Geometry check sheet. Reference: drawing and pictorial views, mm from the part's lowest x, y, z. A direction names the side the tool comes from. Coordinates: 2 decimals unless noted, no trailing zeros. Loops run counter-clockwise (first coordinate to the right, second up) from the corner with the lowest first, then second, coordinate; pieces in that order, holes last. Notation, with made-up numbers: (15.25, 50.25) - (71.25, 50.25) arc R19 cw to (71.25, 71.25) - close; hole circle Ø1 at (-12.75, 8). An arc over 180 degrees is marked (long way). One line per item, written item: value.
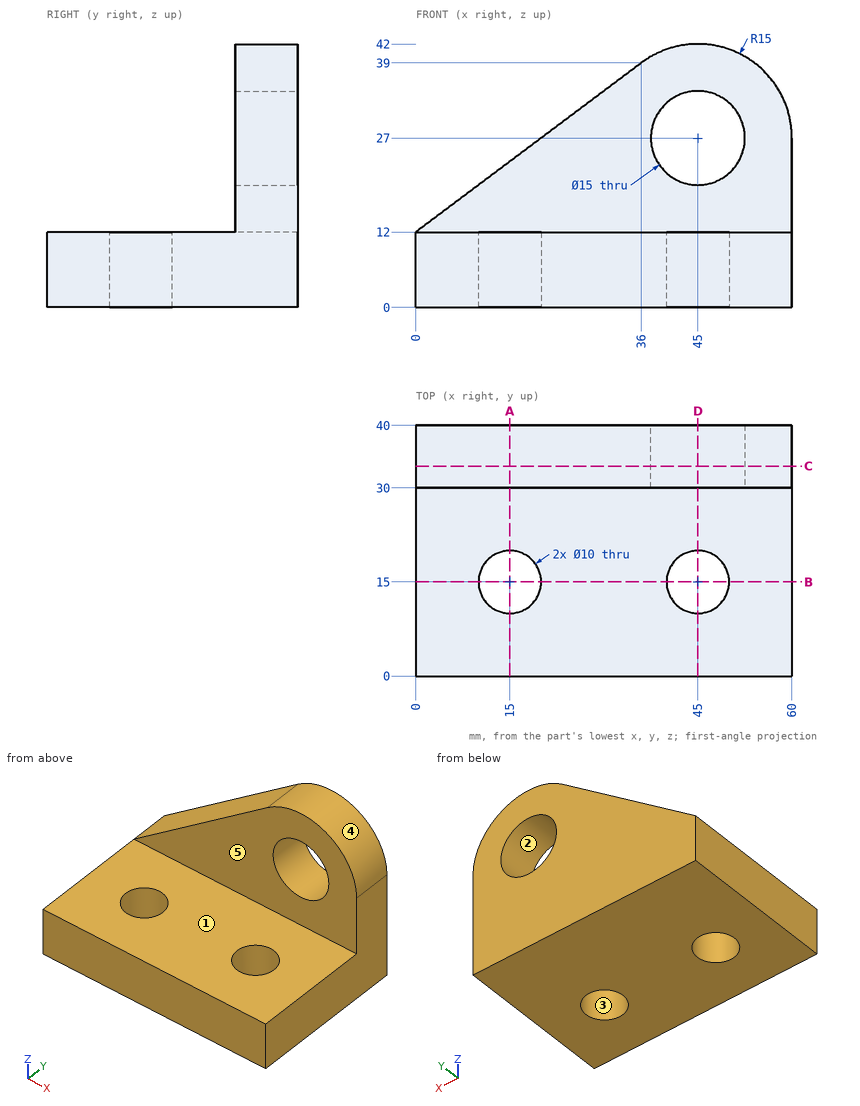
(1) Cross-section at C-C on y = 33.5. Record the cut outline in (x, z), and give its area (3 significant figures).
Reply:
outline: (0, 0) - (60, 0) - (60, 27) arc R15 ccw to (36, 39) - (0, 12) - close; hole circle Ø15 at (45, 27)
area: 1,690 mm2
(2) Access from +Z, -Z, +X, -X, +Y, -Y to the whole of each face (thin tool, end or side, straight path). Record for the marked faces 1 and 2.
Reply:
face 1: +Z, +X, -X, -Y
face 2: +Y, -Y
(3) Cross-section at D-D on x = 45. Record the cut outline in (y, z), and give its area (3 significant figures).
Reply:
outline: (0, 0) - (10, 0) - (10, 12) - (0, 12) - close; (20, 0) - (40, 0) - (40, 19.5) - (30, 19.5) - (30, 12) - (20, 12) - close; (30, 34.5) - (40, 34.5) - (40, 42) - (30, 42) - close
area: 510 mm2
(4) Release check for a two-part mould opening along X. For the marked faces 3, 4 and 5 record: pulls with the +X half, pulls with the -X half, needs draft (parallel to the pull), parting line crosses it, or undercut.
Reply:
face 3: undercut
face 4: parting line crosses it
face 5: needs draft
(5) Go/stop test with flat-tipped pins: pin 1 Ø9 at (x, z) = (45, 27) entering from +Y; pin 2 Ø2 at (y, z) = (29.5, 34.5) entering from -X; pin 3 Ø24 at (x, y) = (26, 20.5) entering from +Z; pin 4 Ø15 at (x, z) = (42.5, 21.5) entering from -Y. Record where each tip stops, or that it passes through.
Reply:
pin 1: through
pin 2: x = 28.85
pin 3: z = 37
pin 4: y = 30
(6) Material ranges on probe 1 along Y at (x, z) = (15, 7); probe 2 along Z at (x, y) = (45, 36); probe 3 along Y at (x, z) = (48, 39), recorded low to high. Write a range as from..to.
Reply:
probe 1: 0..10, 20..40
probe 2: 0..19.5, 34.5..42
probe 3: 30..40
(7) Cross-section at A-A on x = 15. Record the cut outline in (y, z).
Reply:
outline: (0, 0) - (10, 0) - (10, 12) - (0, 12) - close; (20, 0) - (40, 0) - (40, 23.25) - (30, 23.25) - (30, 12) - (20, 12) - close
(8) Cross-section at B-B on y = 15. Record the cut outline in (x, z).
Reply:
outline: (0, 0) - (10, 0) - (10, 12) - (0, 12) - close; (20, 0) - (40, 0) - (40, 12) - (20, 12) - close; (50, 0) - (60, 0) - (60, 12) - (50, 12) - close
